```python
from build123d import *

# Parameters (mm, degrees)
SKETCH1_W             = 90
SKETCH1_H             = 60
BOSS_EXTRUDE1_DEPTH   = 7
M20_CLEARANCE_SLOT1_D = 22
M8_CLEARANCE_SLOT1_D  = 9
SKETCH8_R             = 4.8
CUT_EXTRUDE1_DEPTH    = 7


with BuildPart() as part:
    # Sketch1 → Boss-Extrude1 (new body)
    with BuildSketch(Plane(origin=(0, 0, 0), x_dir=(1, 0, 0), z_dir=(0, 1, 0))):
        with Locations((45, 30)):
            Rectangle(SKETCH1_W, SKETCH1_H)
    extrude(amount=BOSS_EXTRUDE1_DEPTH)

    # M20 Clearance Slot1 (through all)
    with Locations(Plane(origin=(0, 7, 0), x_dir=(1, 0, 0), z_dir=(0, 1, 0))):
        with Locations((25, 30), (65, 30)):
            Hole(M20_CLEARANCE_SLOT1_D / 2)

    # M8 Clearance Slot1 (through all)
    with Locations(Plane(origin=(0, 7, 0), x_dir=(1, 0, 0), z_dir=(0, 1, 0))):
        with Locations((80, 50), (10, 10)):
            Hole(M8_CLEARANCE_SLOT1_D / 2)

    # Sketch8 → Cut-Extrude1 (cut)
    with BuildSketch(Plane(origin=(0, 7, 0), x_dir=(1, 0, 0), z_dir=(0, 1, 0))):
        with Locations(Location((10, 50, 0), (0, 0, 270))):
            Circle(SKETCH8_R)
    extrude(amount=-CUT_EXTRUDE1_DEPTH, mode=Mode.SUBTRACT)


solid = part.part
```
The listing builds one solid part. Answer for the finished solid, in the listing's coordinates (mm). Coordinates: 2 decimals unless noted, no trailing zeros. Loops run counter-clockwise (first coordinate to the right, second up) from the corner with the lowest first, then second, coordinate; pieces in that order, holes last. Notation, with made-up numbers: (66.25, -10) - (85.25, -10) arc R10 ccw to (85.25, 8) - close; hole circle Ø5 at (44.25, 69.25). An arc over 180 degrees is marked (long way). Use a Markdown table: item, result. Add a question column.
1) The part is cut by section A-A, the plane z = -30. Give the vertices of the cut face in (x, y).
2) The mould has two halves that part along Z. Classify faces 1 (the flat face through (44, 3, -60)), 2 (the cylindrical face through (19.924, 3.451, -20.241)), 3 (the flat face through (44, 0, -30)): released by +Z, released by -Z, zero draft, split by the parting line, or undercut.
3) The part is cut by section C-C, the plane z = -10. Give the vertices of the cut face in (x, y).
4) Find the intervals of material crossed by line 1 (X direction, y = 5, z = -50); line 2 (Z direction, x = 25, y = 5.75); line 3 (X direction, y = 4.5, z = -37.5), in increasing order.
5) Given pin 1 (1.5 mm diameter, centred on y = 5, z = -29.5, fed in from -X), flat-ended and moving along its own axis, determine where the tip first touches the part or whether it passes through.
6) The part is cut by section B-B, the plane x = 10. Give the vertices of the cut face in (y, z).
7) The part is cut by section D-D, the plane y = 2.75. Give the vertices of the cut face in (x, z), and give its area (3 significant figures).
Here are the results:
| question | item | result |
|---|---|---|
| 1 | outline | (0, 0) - (14, 0) - (14, 7) - (0, 7) - close; (36, 0) - (54, 0) - (54, 7) - (36, 7) - close; (76, 0) - (90, 0) - (90, 7) - (76, 7) - close |
| 2 | face 1 | released by -Z |
| 2 | face 2 | undercut |
| 2 | face 3 | zero draft |
| 3 | outline | (0, 0) - (5.5, 0) - (5.5, 7) - (0, 7) - close; (14.5, 0) - (90, 0) - (90, 7) - (14.5, 7) - close |
| 4 | line 1 | x = 0 to 5.2, 14.8 to 75.5, 84.5 to 90 |
| 4 | line 2 | z = -60 to -41, -19 to 0 |
| 4 | line 3 | x = 0 to 16.95, 33.05 to 56.95, 73.05 to 90 |
| 5 | pin 1 | stops at x = 0 |
| 6 | outline | (0, -60) - (7, -60) - (7, -54.8) - (0, -54.8) - close; (0, -45.2) - (7, -45.2) - (7, -14.5) - (0, -14.5) - close; (0, -5.5) - (7, -5.5) - (7, 0) - (0, 0) - close |
| 7 | outline | (0, -60) - (90, -60) - (90, 0) - (0, 0) - close; hole circle Ø9.6 at (10, -50); hole circle Ø9 at (10, -10); hole circle Ø22 at (25, -30); hole circle Ø22 at (65, -30); hole circle Ø9 at (80, -50) |
| 7 | area | 4,440 mm^2 |
